from build123d import *

# Parameters (mm, degrees)
SKETCH_1_R      = 2
EXTRUDE_1_DEPTH = 23
SKETCH_2_R      = 4
EXTRUDE_2_DEPTH = 2
CHAMFER_1_SIZE  = 0.2


with BuildPart() as part:
    # 草图1 → 拉伸1 (new body)
    with BuildSketch(Plane.XY):
        Circle(SKETCH_1_R)
    extrude(amount=EXTRUDE_1_DEPTH)

    # 草图2 → 拉伸2 (add)
    with BuildSketch(Plane(origin=(0, 0, 0), x_dir=(-1, 0, 0), z_dir=(0, 0, -1))):
        Circle(SKETCH_2_R)
    extrude(amount=EXTRUDE_2_DEPTH)

    # 倒角1
    chamfer_1_edges = [part.edges().sort_by_distance(p)[0] for p in [
        (-2, 0, 23),
    ]]
    chamfer(chamfer_1_edges, length=CHAMFER_1_SIZE)


solid = part.part
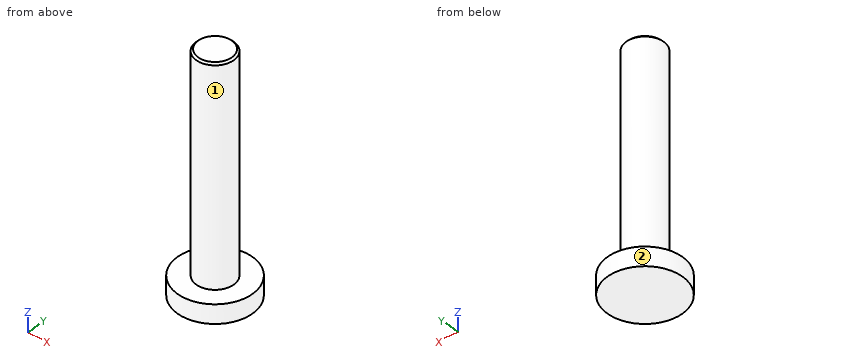
Check sheet for the modelled part. Datum: model origin and axes. Units: mm. Face numbers are marked on the shaded views. A direction names the side the tool comes from. Round coordinates to 2 decimals unless told otherwise and drop trailing zeros. Loops run counter-clockwise (first coordinate to the right, second up) from the corner with the lowest first, then second, coordinate; pieces in that order, holes last.
1. Sectioned sample at C-C on z = 18.25. Record the boundary of the cut face in (x, y), and give its area (3 significant figures).
2. Gauge pin test, flat ends, axial feed: pin 1 Ø3 at (x, z) = (2, 12) entering from +Y; pin 2 Ø3 at (y, z) = (0.5, 7.5) entering from +X; pin 3 Ø2 at (y, z) = (-0.5, 4) entering from -X. Record the tip position at first contact, or that the pin passes through.
3. Sectioned sample at A-A on y = 0. Record the boundary of the cut face in (x, z).
4. Sectioned sample at D-D on x = -2.5. Record the boundary of the cut face in (y, z), and give its area (3 significant figures).
5. Set-up check for the marked faces 1 and 2: record each of +Z, -Z, +X, -X, +Y, -Y from which the full face is reachable in a straight line by a thin tool's end or side.
6. Scan lines: probe 1 along Z at (x, y) = (-1, -2.25); probe 2 along Y at (x, z) = (-0.75, 6.5); probe 3 along X at (y, z) = (1, 5). Record each from-to range of solid material in increasing order.
Recorded:
1. outline: circle Ø4 at (0, 0)
1. area: 12.6 mm2
2. pin 1: stops at y = 1.94
2. pin 2: stops at x = 2
2. pin 3: stops at x = -2
3. outline: (-4, -2) - (4, -2) - (4, 0) - (2, 0) - (2, 22.8) - (1.8, 23) - (-1.8, 23) - (-2, 22.8) - (-2, 0) - (-4, 0) - close
4. outline: (-3.12, -2) - (3.12, -2) - (3.12, 0) - (-3.12, 0) - close
4. area: 12.5 mm2
5. face 1: +Z
5. face 2: +Z, -Z
6. probe 1: z = -2 to 0
6. probe 2: y = -1.85 to 1.85
6. probe 3: x = -1.73 to 1.73
